For this review, take the finished solid that the model builds, in its own axes (mm). A direction names the side the tool comes from. Give positions to 0.01 mm unless a question says otherwise; leave off trailing zeros. Order: outer loops, then holes, each group sorted by start corner. A loop starts at its lowest first (then second) coordinate and runs counter-clockwise, first axis right, second up. Notation, with made-up numbers: (60, -19.75) - (94, -19.75) arc R19 cw to (94, -3.75) - close; hole circle Ø8 at (48, 10). An arc over 180 degrees is marked (long way). One line per item, written item: value.
```python
from build123d import *


with BuildPart() as part:
    # Sketch → Revolution (revolve)
    with BuildSketch(Plane.XZ):
        with BuildLine():
            Line((-13.7, 41.2), (-13.7, 34.2))
            Line((-13.7, 34.2), (-18.2, 34.2))
            Line((-18.2, 34.2), (-18.2, 35.8))
            Line((-18.2, 35.8), (-16.2, 35.8))
            Line((-16.2, 35.8), (-16.2, 38.2))
            Line((-22.5, 38.2), (-16.2, 38.2))
            ThreePointArc((-23.5, 39.2), (-23.207107, 38.492893), (-22.5, 38.2))
            Line((-23.5, 39.2), (-23.5, 41.2))
            ThreePointArc((-21.5, 43.2), (-22.914214, 42.614214), (-23.5, 41.2))
            Line((-21.5, 43.2), (21.5, 43.2))
            ThreePointArc((23.5, 41.2), (22.914214, 42.614214), (21.5, 43.2))
            Line((23.5, 41.2), (23.5, 39.2))
            ThreePointArc((22.5, 38.2), (23.207107, 38.492893), (23.5, 39.2))
            Line((16.2, 38.2), (22.5, 38.2))
            Line((16.2, 35.8), (16.2, 38.2))
            Line((18.2, 35.8), (16.2, 35.8))
            Line((18.2, 34.2), (18.2, 35.8))
            Line((13.7, 34.2), (18.2, 34.2))
            Line((13.7, 41.2), (13.7, 34.2))
            Line((13.7, 41.2), (-13.7, 41.2))
        make_face()
    revolve(axis=Axis((0, 0, 0), (1, 0, 0)))


solid = part.part
```
(1) Wall thickness on line 1 (Z direction, x = -16.25, y = 0); line 2 (Z direction, x = -16.15, y = 0): over which ranges is each line inside the solid? List them lowest first. Write a range as from..to.
Answers below:
line 1: z = -43.2..-38.2, -35.8..-34.2, 34.2..35.8, 38.2..43.2
line 2: z = -43.2..-34.2, 34.2..43.2
(2) Take a section at B-B (x = -9.5). Write out the cut boundary in (y, z).
Answers below:
outline: circle Ø86.4 at (0, 0); hole circle Ø82.4 at (0, 0)
(3) For P1, Ø6, axis at y = -23.5, z = -17.5, coming from the -X side; P2, Ø1.5, axis at x = 16.5, z = 24.5, coming from the -Y side; P3, Ø5, axis at x = 12.5, z = 14.5, coming from the +Y side; P4, Ø2, axis at x = -17.5, y = -29.5, coming from the -Z side, all flat-tipped, find the tip position at first contact; note any pin that passes through.
Answers below:
P1: passes through
P2: stops at y = -36.09
P3: stops at y = 41.5
P4: stops at z = -32.47
(4) Take a section at A-A (x = 15). Write out the cut boundary in (y, z).
Answers below:
outline: circle Ø86.4 at (0, 0); hole circle Ø68.4 at (0, 0)
(5) Draft analysis for pull direction Y (two halves, no side actions). For faces 1 (the face through (23.5, 36.4, 15.1)), 2 (the face through (17.186, 21.784, -28.41)), 3 (the face through (0.301, 42.173, -9.365)), state which applies: pulls with the +Y half, pulls with the -Y half, needs draft (parallel to the pull), parting line crosses it, or undercut.
Answers below:
face 1: needs draft
face 2: undercut
face 3: parting line crosses it
(6) Machinability: for faces 4 (the face through (18.2, 13, -32)), 5 (the face through (-17.186, 21.784, -28.41)), 6 (the face through (-0.192, -12.375, 39.297)), 7 (the face through (-23.5, 36.4, -15.1)), 8 (the face through (15.98, -10.27, 32.62)), which of the approach directions +Z, -Z, +X, -X, +Y, -Y give a long, thin tool a straight path to every point of the face, cutting with its end or side? Answer none if there is none.
Answers below:
face 4: +X
face 5: -X
face 6: none
face 7: +Z, -Z, -X, +Y, -Y
face 8: +X, -X
